```python
from build123d import *

# Parameters (mm, degrees)
SALIENTE_EXTRUIR1_DEPTH = 5
CROQUIS2_R              = 27.5
CORTAR_EXTRUIR1_DEPTH   = 10


with BuildPart() as part:
    # Croquis1 → Saliente-Extruir1 (new body)
    with BuildSketch(Plane.XY):
        Polygon((0, 215), (0, 0), (246, 0), (246, 145), (216, 145), (216, 185), (176, 185), (176, 215), align=None)
        Polygon((-246, 145), (-246, 0), (0, 0), (0, 215), (-176, 215), (-176, 185), (-216, 185), (-216, 145), align=None)
        Polygon((0, 0), (-246, 0), (-246, -145), (-216, -145), (-216, -185), (-176, -185), (-176, -215), (176, -215), (176, -185), (216, -185), (216, -145), (246, -145), (246, 0), align=None)
    extrude(amount=SALIENTE_EXTRUIR1_DEPTH)

    # Croquis2 → Cortar-Extruir1 (cut)
    with BuildSketch(Plane.XY.offset(5)):
        with Locations((-180, -107)):
            Circle(CROQUIS2_R)
        with Locations((0, -107)):
            Circle(CROQUIS2_R)
        with Locations((180, -107)):
            Circle(CROQUIS2_R)
    extrude(amount=-CORTAR_EXTRUIR1_DEPTH, mode=Mode.SUBTRACT)


solid = part.part
```
Design review of the part built by this model. Coordinates are the model's own, in mm. Coordinates: 2 decimals unless noted, no trailing zeros. Write each loop counter-clockwise with the first axis right and the second up, starting at its lowest first coordinate (ties: lowest second). Pieces come first, ordered by that corner, then holes. Notation, with made-up numbers: M 4.5,61.5 L 57.5,61.5 A14 cw 57.5,70.5 Z; hole C 32.5,59.25 d7. An arc over 180 degrees is marked long. Answer as a JSON object with one key per item and string values.
Item 1: Add section B-B, the plane y = -107. Give the boundary of the cut face in (x, z).
Outcome:
{"outline": "M -246,0 L -207.5,0 L -207.5,5 L -246,5 Z; M -152.5,0 L -27.5,0 L -27.5,5 L -152.5,5 Z; M 27.5,0 L 152.5,0 L 152.5,5 L 27.5,5 Z; M 207.5,0 L 246,0 L 246,5 L 207.5,5 Z"}
Item 2: Insertion check: pin 1 Ø1.5 at (y, z) = (-206.5, 3.5) entering from -X; pin 2 Ø1.5 at (y, z) = (-200, 3.5) entering from +X; pin 3 Ø1.5 at (x, z) = (-197.5, 3.5) entering from +Y. Each pin has a flat end and moves straight along its axis. Give the tip position at first contact, or say it passes through.
Outcome:
{"pin 1": "x = -176", "pin 2": "x = 176", "pin 3": "y = 185"}
Item 3: Add section D-D, the plane y = 168. Give the boundary of the cut face in (x, z).
Outcome:
{"outline": "M -216,0 L 216,0 L 216,5 L -216,5 Z"}
Item 4: Add section A-A, the plane x = 0. Give the boundary of the cut face in (y, z), and give its area (4 significant figures).
Outcome:
{"outline": "M -215,0 L -134.5,0 L -134.5,5 L -215,5 Z; M -79.5,0 L 215,0 L 215,5 L -79.5,5 Z", "area": "1,875 mm²"}
Item 5: Draft analysis for pull direction X (two halves, no side actions). For faces 1 (the cylindrical face through (-153.77, -98.74, 2.54)), 2 (the flat face through (-3, 3, 5)), state which applies: pulls with the +X half, pulls with the -X half, needs draft (parallel to the pull), parting line crosses it, or undercut.
Outcome:
{"face 1": "undercut", "face 2": "needs draft"}
Item 6: Add section C-C, the plane z = 1.2. Give the boundary of the cut face in (x, y), and give its area (3 significant figures).
Outcome:
{"outline": "M -246,-145 L -216,-145 L -216,-185 L -176,-185 L -176,-215 L 176,-215 L 176,-185 L 216,-185 L 216,-145 L 246,-145 L 246,145 L 216,145 L 216,185 L 176,185 L 176,215 L -176,215 L -176,185 L -216,185 L -216,145 L -246,145 Z; hole C -180,-107 d55; hole C 0,-107 d55; hole C 180,-107 d55", "area": "191,000 mm²"}
Item 7: Wall thickness on probe 1 along Y at (x, z) = (-180, 1.3); probe 2 along Y at (x, z) = (0, 2.45); probe 3 along X at (y, z) = (-149.5, 3.65): over which ranges is each line inside the solid? List them lowest first.
Outcome:
{"probe 1": "-185 to -134.5, -79.5 to 185", "probe 2": "-215 to -134.5, -79.5 to 215", "probe 3": "-216 to 216"}
